```python
from build123d import *

# Parameters (mm, degrees)
F1_DEPTH = 12.6
F2_COUNT = 12
F3_R     = 6.1544610685
F4_DEPTH = 25


with BuildPart() as f1:
    # F0 (on Front) → F1 (new body)
    with BuildSketch(Plane.XZ):
        with BuildLine():
            ThreePointArc((2.7852032442, 25.3538235305), (-10.8298302985, -21.3004259569), (33.3673953593, -1.0867331287))
            ThreePointArc((33.3673953593, -1.0867331287), (26.8600881876, 16.3894925292), (10.5075874745, 25.3538235305))
            ThreePointArc((10.5075874745, 25.3538235305), (8.9226743944, 25.5371357629), (7.3296460588, 25.6255301502))
            ThreePointArc((7.3296460588, 25.6255301502), (5.0516276545, 25.5866348058), (2.7852032442, 25.3538235305))
        make_face()
        with BuildLine():
            ThreePointArc((7.3296460588, 25.6255301502), (8.9226743944, 25.5371357629), (10.5075874745, 25.3538235305))
            ThreePointArc((10.5075874745, 25.3538235305), (10.6097622585, 27.8798441888), (10.28181369, 30.3865691018))
            ThreePointArc((10.28181369, 30.3865691018), (9.4245102455, 33.0410725411), (8.0713397316, 35.4803936077))
            ThreePointArc((8.0713397316, 35.4803936077), (6.6463953593, 33.6211668014), (5.2214509871, 35.4803936077))
            ThreePointArc((5.2214509871, 35.4803936077), (3.8682804732, 33.0410725411), (3.0109770287, 30.3865691018))
            ThreePointArc((3.0109770287, 30.3865691018), (2.6830284602, 27.8798441888), (2.7852032442, 25.3538235305))
            ThreePointArc((2.7852032442, 25.3538235305), (5.0516276545, 25.5866348058), (7.3296460588, 25.6255301502))
        make_face()
    extrude(amount=F1_DEPTH)

    # F2: F1 ×12 about axis
    f2_axis = Axis((6.6463953593, 0, -1.0867331287), (0, 1, 0))


with BuildPart() as f1_1:
    add(f1.part)
    for i in range(1, F2_COUNT):
        add(f1.part.rotate(f2_axis, i * 360 / F2_COUNT))

    # F3 (on face) → F4 (cut)
    with BuildSketch(Plane.XZ.offset(12.6)):
        with Locations((6.6463953593, -1.0867331287)):
            Circle(F3_R)
    extrude(amount=-F4_DEPTH, mode=Mode.SUBTRACT)


solid = f1_1.part
```
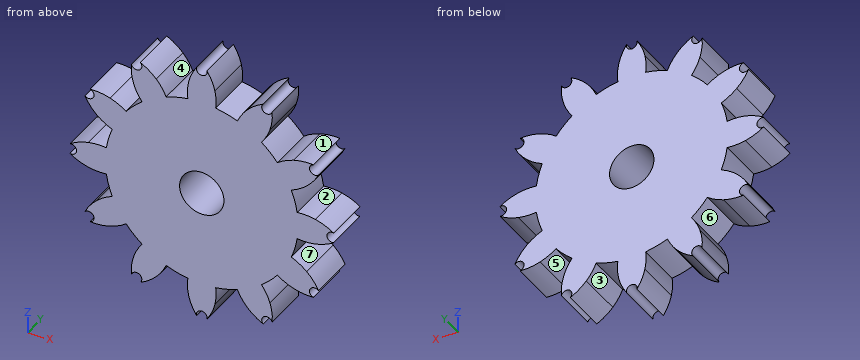
Verification items for the finished model (mm, model axes). Face numbers are marked on the shaded views. A direction names the side the tool comes from. Give positions to 0.01 mm unless a question says otherwise; leave off trailing zeros. Order: outer loops, then holes, each group sorted by start corner. A loop starts at its lowest first (then second) coordinate and runs counter-clockwise, first axis right, second up. Notation, with made-up numbers: M 5.5,12 L 11.5,12 A13 ccw 11.5,20 Z; hole C 2,-27.75 d8. An arc over 180 degrees is marked long. Return JSON: item names as keys, results as strings. Group by question number.
1) Section check D-D on x = 15.5. Record the cut outline in (y, z), and give its area (3 significant figures).
2) Mould release check, pull along Z, two halves, no side actions. Record for the marked faces 1, 2 and 3: pulls with the +Z half, pulls with the -Z half, needs draft (parallel to the pull), parting line crosses it, or undercut.
3) Section check A-A on z = 27. Record the cut outline in (x, y).
4) Scan lines: line 1 (Z direction, x = 36, y = -10); line 2 (Z direction, x = -22, y = -8); line 3 (X direction, y = -3.5, z = -30). Record each from-to range of solid material in increasing order.
5) Go/stop test with flat-tipped pins: pin 1 Ø2.5 at (x, z) = (37.98, 17.01) entering from +Y; pin 2 Ø8 at (x, z) = (-13.5, 2.5) entering from +Y; pin 3 Ø1 at (y, z) = (-1.5, -8) entering from +X; pin 4 Ø6 at (x, y) = (-10.5, -1.5) entering from +Z. Record where each tip stops, or that it passes through.
6) Section check B-B on x = 4. Record the cut outline in (y, z), and give its area (3 significant figures).
7) Section check C-C on z = 4. Record the cut outline in (x, y).
8) Access from +Z, -Z, +X, -X, +Y, -Y to the whole of each face (thin tool, end or side, straight path). Record for the marked faces 4, 5, 6 and 7.
Answer block:
{
 "1": {"outline": "M -12.6,-26.3 L 0,-26.3 L 0,24.12 L -12.6,24.12 Z", "area": "635 mm^2"},
 "2": {"face 1": "pulls with the +Z half", "face 2": "undercut", "face 3": "pulls with the -Z half"},
 "3": {"outline": "M -12.81,-12.6 L -5.12,-12.6 L -5.12,0 L -12.81,0 Z; M 2.67,-12.6 L 10.62,-12.6 L 10.62,0 L 2.67,0 Z; M 18.41,-12.6 L 26.11,-12.6 L 26.11,0 L 18.41,0 Z"},
 "4": {"line 1": "z = -20.64 to -13.94, -5.03 to 2.85, 11.76 to 18.47", "line 2": "z = -20.6 to -13.3, -5.06 to 2.89, 11.13 to 18.43", "line 3": "x = -12.89 to -5.8, 2.68 to 10.61, 19.09 to 26.18"},
 "5": {"pin 1": "passes through", "pin 2": "stops at y = 0", "pin 3": "stops at x = 32.59", "pin 4": "stops at z = 31.29"},
 "6": {"outline": "M -12.6,-35.51 L 0,-35.51 L 0,-6.64 L -12.6,-6.64 Z; M -12.6,4.47 L 0,4.47 L 0,33.34 L -12.6,33.34 Z", "area": "727 mm^2"},
 "7": {"outline": "M -19.59,-12.6 L 3.18,-12.6 L 3.18,0 L -19.59,0 Z; M 10.11,-12.6 L 32.88,-12.6 L 32.88,0 L 10.11,0 Z"},
 "8": {"face 4": "+Z, +Y, -Y", "face 5": "-Z, +Y, -Y", "face 6": "+Y, -Y", "face 7": "+X, +Y, -Y"}
}
